Source: CAD feature listing. Evaluate the final solid. Frame: model axes, mm. Give positions to 0.01 mm unless a question says otherwise; leave off trailing zeros. Order: outer loops, then holes, each group sorted by start corner. A loop starts at its lowest first (then second) coordinate and runs counter-clockwise, first axis right, second up. Notation, with made-up numbers: (65, 86) - (91, 86) arc R27 ccw to (91, 124) - close; hole circle Ø1 at (46.25, 61.5). An arc over 180 degrees is marked (long way). Use CSV: the item, a comma, the result in double quotes.
```python
from build123d import *

# Parameters (mm, degrees)
SKETCH1_R           = 22.5
BOSS_EXTRUDE1_DEPTH = 1.6
SKETCH2_R           = 0.429187569
CUT_EXTRUDE1_DEPTH  = 32.860006277


with BuildPart() as part:
    # Sketch1 → Boss-Extrude1 (new body)
    with BuildSketch(Plane(origin=(0, 0, 0), x_dir=(1, 0, 0), z_dir=(0, 1, 0))):
        with Locations(Location((0, 0, 0), (0, 0, 270))):
            Circle(SKETCH1_R)
    extrude(amount=BOSS_EXTRUDE1_DEPTH)

    # Sketch2 → Cut-Extrude1 (cut, through all)
    with BuildSketch(Plane.XZ):
        with Locations(Location((9.721005352, 11.34055894, 0), (0, 0, 270))):
            Circle(SKETCH2_R)
        with Locations(Location((7.181005352, 11.34055894, 0), (0, 0, 270))):
            Circle(SKETCH2_R)
        with Locations(Location((4.641005352, 11.34055894, 0), (0, 0, 270))):
            Circle(SKETCH2_R)
        with Locations(Location((2.101005352, 11.34055894, 0), (0, 0, 270))):
            Circle(SKETCH2_R)
        with Locations(Location((-0.438994648, 11.34055894, 0), (0, 0, 270))):
            Circle(SKETCH2_R)
        with Locations(Location((-2.978994648, 11.34055894, 0), (0, 0, 270))):
            Circle(SKETCH2_R)
        with Locations(Location((-5.518994648, 11.34055894, 0), (0, 0, 270))):
            Circle(SKETCH2_R)
        with Locations(Location((-8.058994648, 11.34055894, 0), (0, 0, 270))):
            Circle(SKETCH2_R)
        with Locations(Location((9.721005352, -11.469960564, 0), (0, 0, 270))):
            Circle(SKETCH2_R)
        with Locations(Location((7.181005352, -11.469960564, 0), (0, 0, 270))):
            Circle(SKETCH2_R)
        with Locations(Location((4.641005352, -11.469960564, 0), (0, 0, 270))):
            Circle(SKETCH2_R)
        with Locations(Location((2.101005352, -11.469960564, 0), (0, 0, 270))):
            Circle(SKETCH2_R)
        with Locations(Location((-0.438994648, -11.469960564, 0), (0, 0, 270))):
            Circle(SKETCH2_R)
        with Locations(Location((-2.978994648, -11.469960564, 0), (0, 0, 270))):
            Circle(SKETCH2_R)
        with Locations(Location((-5.518994648, -11.469960564, 0), (0, 0, 270))):
            Circle(SKETCH2_R)
        with Locations(Location((-8.058994648, -11.469960564, 0), (0, 0, 270))):
            Circle(SKETCH2_R)
        with Locations(Location((-8.554850814, 3.728315564, 0), (0, 0, 270))):
            Circle(SKETCH2_R)
        with Locations(Location((-8.554850814, 1.188315564, 0), (0, 0, 270))):
            Circle(SKETCH2_R)
        with Locations(Location((-8.554850814, -1.351684436, 0), (0, 0, 270))):
            Circle(SKETCH2_R)
        with Locations(Location((-8.554850814, -3.891684436, 0), (0, 0, 270))):
            Circle(SKETCH2_R)
        with Locations(Location((-3.513785175, 6.72628012, 0), (0, 0, 270))):
            Circle(SKETCH2_R)
        with Locations(Location((-14.013865652, 15.451077266, 0), (0, 0, 270))):
            Circle(SKETCH2_R)
        with Locations(Location((-18.940700894, 8.847549383, 0), (0, 0, 270))):
            Circle(SKETCH2_R)
        with Locations(Location((-3.513785175, -3.436577571, 0), (0, 0, 270))):
            Circle(SKETCH2_R)
        with Locations(Location((-8.884144238, -19.158046189, 0), (0, 0, 270))):
            Circle(SKETCH2_R)
        with Locations(Location((-0.906931184, -21.088850712, 0), (0, 0, 270))):
            Circle(SKETCH2_R)
        with Locations(Location((19.722815894, 6.970464171, 0), (0, 0, 270))):
            Circle(SKETCH2_R)
        with Locations(Location((18.971783185, -9.009472345, 0), (0, 0, 270))):
            Circle(SKETCH2_R)
    extrude(amount=-CUT_EXTRUDE1_DEPTH, mode=Mode.SUBTRACT)


solid = part.part
```
Item 1: Section B-B on z = -13.5. Return the cut outline in (x, y), then the cut area to 3 significant figures.
Filled in:
outline,"(-18, 0) - (18, 0) - (18, 1.6) - (-18, 1.6) - close"
area,"57.6 mm2"
Item 2: Section C-C on x = 15.5. Return the cut outline in (y, z).
Filled in:
outline,"(0, -16.31) - (1.6, -16.31) - (1.6, 16.31) - (0, 16.31) - close"
Item 3: Section A-A on y = 0.9. Count the separate pieces of the cut face and the enclosed holes in it, then the cut area to 3 significant figures.
Filled in:
separate pieces,"1"
enclosed holes,"28"
area,"1,570 mm2"
Item 4: Material intervals for line 1 (Z direction, x = 9.5, y = 1.4); line 2 (X direction, y = 0.3, z = 1); line 3 (X direction, y = 1.1, z = 1.5), sorted ascending. Write a range as from..to.
Filled in:
line 1,"z = -20.4..-11.84, -11.1..10.97, 11.71..20.4"
line 2,"x = -22.48..-8.94, -8.17..22.48"
line 3,"x = -22.45..-8.85, -8.26..22.45"
